Work out the finished part from the listing and answer in its coordinate system (mm). Face numbers are marked on the shaded views. A direction names the side the tool comes from. Round coordinates to 2 decimals unless told otherwise and drop trailing zeros. Loops run counter-clockwise (first coordinate to the right, second up) from the corner with the lowest first, then second, coordinate; pieces in that order, holes last. Notation, with made-up numbers: (81, 20.25) - (96, 20.25) arc R10 cw to (96, 34.25) - close; hole circle Ø9 at (7, 45.25). An arc over 180 degrees is marked (long way). Answer as CSV lines item,"result". Start each with the question number.
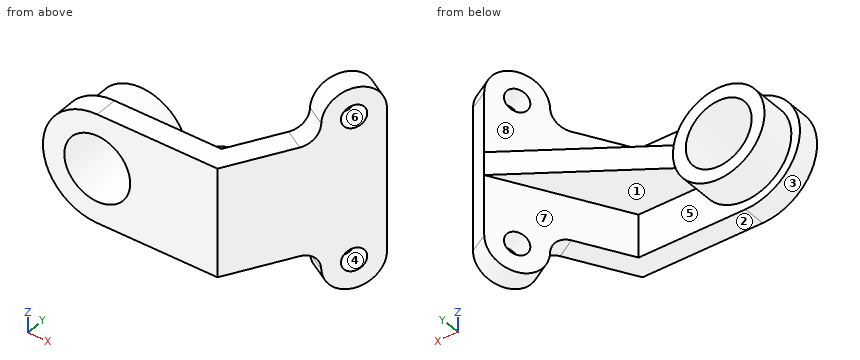
```python
from build123d import *

# Parameters (mm, degrees)
SKETCH_1_R      = 32
EXTRUDE_1_DEPTH = 16
SKETCH_1_3_R    = 32
SKETCH_1_3_R_2  = 23
EXTRUDE_2_DEPTH = 41
SKETCH_3_R      = 8
EXTRUDE_3_DEPTH = 16
RIB_1_REACH     = 182.854
SKETCH_4_WALL_W = 471.13581316
SKETCH_4_WALL_H = 16


with BuildPart() as part:
    # Sketch 1 → Extrude 1 (new body)
    with BuildSketch(Plane(origin=(0, 0, 0), x_dir=(1, 0, 0), z_dir=(0, 1, 0))):
        with BuildLine():
            Line((0, 38), (84, 38))
            Line((84, 38), (84, -38))
            Line((84, -38), (0, -38))
            ThreePointArc((0, -38), (-38, 0), (0, 38))
        make_face()
        with Locations(Location((0, 0, 0), (0, 0, 270))):
            Circle(SKETCH_1_R, mode=Mode.SUBTRACT)
    extrude(amount=EXTRUDE_1_DEPTH)

    # Sketch 1_3 → Extrude 2 (add)
    with BuildSketch(Plane(origin=(0, 0, 0), x_dir=(1, 0, 0), z_dir=(0, 1, 0))):
        with Locations(Location((0, 0, 0), (0, 0, 270))):
            Circle(SKETCH_1_3_R)
        with Locations(Location((0, 0, 0), (0, 0, 270))):
            Circle(SKETCH_1_3_R_2, mode=Mode.SUBTRACT)
    extrude(amount=EXTRUDE_2_DEPTH)

    # Sketch 3 → Extrude 3 (add)
    with BuildSketch(Plane(origin=(63, -36.373066959, 0), x_dir=(0, 0, 1), z_dir=(-0.8660254037844398, 0.499999999999998, 0))):
        with BuildLine():
            Line((-38, 42), (-38, 92))
            ThreePointArc((-38, 92), (-41.807611845, 101.192388155), (-51, 105))
            Line((-51, 105), (-50, 105))
            ThreePointArc((-50, 105), (-70, 125), (-50, 145))
            Line((-50, 145), (50, 145))
            ThreePointArc((50, 145), (70, 125), (50, 105))
            Line((50, 105), (51, 105))
            ThreePointArc((51, 105), (41.807611845, 101.192388155), (38, 92))
            Line((38, 92), (38, 42))
            Line((38, 42), (-38, 42))
        make_face()
        with Locations(Location((-50, 125, 0), (0, 0, 270))):
            Circle(SKETCH_3_R, mode=Mode.SUBTRACT)
        with Locations(Location((50, 125, 0), (0, 0, 90))):
            Circle(SKETCH_3_R, mode=Mode.SUBTRACT)
    extrude(amount=EXTRUDE_3_DEPTH)

    # Sketch 4 wall → Rib 1 (add, up to next)
    with BuildSketch(Plane(origin=(76.821796769, 67.600308295, 0), x_dir=(-0.834455975571, -0.551074609136, 0), z_dir=(0.551074609136, -0.834455975571, 0)), mode=Mode.PRIVATE) as rib_1_sk1:
        Rectangle(SKETCH_4_WALL_W, SKETCH_4_WALL_H)
    rib_1_tool1 = extrude(rib_1_sk1.sketch, amount=RIB_1_REACH, mode=Mode.PRIVATE) - part.part
    add(rib_1_tool1.solids().sort_by_distance((76.821796769, 67.600308295, 0))[0])


solid = part.part
```
Item 1: Section C-C, the plane z = 47 is taken. Give the vertices of the cut face in (x, y).
Item 2: Section A-A, the plane z = 0 is taken. Give the vertices of the cut face in (x, y).
Item 3: Find the intervals of material crossed by L1, parallel to X at y = 35, z = -11; L2, parallel to Y at x = 21.5, z = 14.5; L3, parallel to Y at x = 122, z = 45, in increasing order.
Item 4: Section B-B, the plane y = 28.5 is taken. Give the vertices of the cut face in (x, z).
Item 5: Flat-ended cylindrical pins translate along their axes: pin 1 Ø5 at (x, y) = (91.5, 60.5) entering from -Z; pin 2 Ø24.5 at (x, y) = (55, 52) entering from +Z; pin 3 Ø5 at (x, y) = (104.5, 34.5) entering from +Z; pin 4 Ø10 at (x, z) = (82, 45.5) entering from +Y. Find the tip coordinate at first contact, or state that the pin passes through.
Item 6: Which of the six approach directions +Z, -Z, +X, -X, +Y, -Y give full straight-line access (tool end or side, diameter ignored) to the marked faces 5, 6, 7 and 8?
Item 7: Section D-D, the plane x = 59 is taken. Give the vertices of the cut face in (y, z).
Item 8: Determine the mould class of the marked faces 1, 2, 3 and 4 for opening direction X: pulls with the +X half, pulls with the -X half, needs draft (parallel to the pull), parting line crosses it, or undercut.
Answer:
1,outline,"(101.33, 62.01) - (115.18, 54.01) - (121.79, 65.46) - (107.94, 73.46) - close; (115.35, 86.3) - (129.21, 78.3) - (135.5, 89.2) - (121.64, 97.2) - close"
2,outline,"(-38, 0) - (-23, 0) - (-23, 41) - (-32, 41) - (-32, 16) - (-38, 16) - close; (23, 0) - (84, 0) - (135.5, 89.2) - (121.64, 97.2) - (32, 38) - (32, 41) - (23, 41) - close"
3,L1,"x = -30.05 to -20.2, 20.2 to 30.05, 85.73 to 104.21"
3,L2,"y = 0 to 41"
3,L3,"y = 65.82 to 66.69, 81.11 to 96.99"
4,outline,"(30.98, -8) - (81.98, -8) - (81.98, -38) - (100.45, -38) - (100.45, 38) - (81.98, 38) - (81.98, 8) - (30.98, 8) arc R32 ccw (long way) to start; hole circle Ø46 at (0, 0)"
5,pin 1,"stops at z = -8"
5,pin 2,"stops at z = 8"
5,pin 3,"stops at z = 38"
5,pin 4,"passes through"
6,face 5,"+Y"
6,face 6,"none"
6,face 7,"-Z, +Y"
6,face 8,"+Z, +Y"
7,outline,"(0, -38) - (16, -38) - (16, -8) - (55.83, -8) - (55.83, 8) - (16, 8) - (16, 38) - (0, 38) - close"
8,face 1,"undercut"
8,face 2,"needs draft"
8,face 3,"pulls with the -X half"
8,face 4,"undercut"
